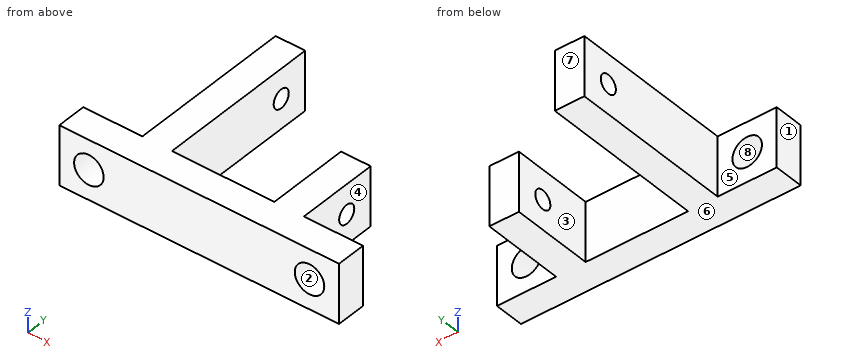
from build123d import *

# Parameters (mm, degrees)
SKETCH1_W           = 22.033357
SKETCH1_H           = 6.35
SKETCH1_W_2         = 12.7
BOSS_EXTRUDE1_DEPTH = 12.7
CUT_EXTRUDE1_REACH  = 49.433
SKETCH2_R           = 2
CUT_EXTRUDE2_REACH  = 8.35
SKETCH3_R           = 3.175
CUT_EXTRUDE3_REACH  = 49.433
SKETCH4_R           = 2


with BuildPart() as part:
    # Sketch1 → Boss-Extrude1 (new body)
    with BuildSketch(Plane.XY):
        Rectangle(SKETCH1_W, SKETCH1_H)
        Polygon((-11.0166785, -3.175), (-11.0166785, 3.175), (-11.0166785, 38.51148), (-17.3666785, 38.51148), (-17.3666785, 3.175), (-17.3666785, -3.175), align=None)
        Polygon((11.0166785, 20.87372), (11.0166785, 3.175), (11.0166785, -3.175), (17.3666785, -3.175), (17.3666785, 3.175), (17.3666785, 20.87372), align=None)
        with Locations((-23.7166785, 0)):
            Rectangle(SKETCH1_W_2, SKETCH1_H)
        with Locations((23.7166785, 0)):
            Rectangle(SKETCH1_W_2, SKETCH1_H)
    extrude(amount=BOSS_EXTRUDE1_DEPTH)

    # Sketch2 → Cut-Extrude1 (cut, up to next)
    with BuildSketch(Plane(origin=(17.3666785, 0, 0), x_dir=(0, 0, -1), z_dir=(1, 0, 0)), mode=Mode.PRIVATE) as cut_extrude1_sk1:
        with Locations((-6.35, 14.52372)):
            Circle(SKETCH2_R)
    cut_extrude1_tool1 = extrude(cut_extrude1_sk1.sketch, amount=-CUT_EXTRUDE1_REACH, mode=Mode.PRIVATE) & part.part
    add(cut_extrude1_tool1.solids().sort_by_distance((17.366678, 14.52372, 6.35))[0], mode=Mode.SUBTRACT)

    # Sketch3 → Cut-Extrude2 (cut, up to next)
    with BuildSketch(Plane(origin=(0, 3.175, 0), x_dir=(1, 0, 0), z_dir=(0, 1, 0)), mode=Mode.PRIVATE) as cut_extrude2_sk1:
        with Locations((-23.7166785, -6.35)):
            Circle(SKETCH3_R)
    cut_extrude2_tool1 = extrude(cut_extrude2_sk1.sketch, amount=-CUT_EXTRUDE2_REACH, mode=Mode.PRIVATE) & part.part
    add(cut_extrude2_tool1.solids().sort_by_distance((-23.716678, 3.175, 6.35))[0], mode=Mode.SUBTRACT)
    # Sketch3 → Cut-Extrude2 (cut, up to next)
    with BuildSketch(Plane(origin=(0, 3.175, 0), x_dir=(1, 0, 0), z_dir=(0, 1, 0)), mode=Mode.PRIVATE) as cut_extrude2_sk2:
        with Locations((23.7166785, -6.35)):
            Circle(SKETCH3_R)
    cut_extrude2_tool2 = extrude(cut_extrude2_sk2.sketch, amount=-CUT_EXTRUDE2_REACH, mode=Mode.PRIVATE) & part.part
    add(cut_extrude2_tool2.solids().sort_by_distance((23.716679, 3.175, 6.35))[0], mode=Mode.SUBTRACT)

    # Sketch4 → Cut-Extrude3 (cut, up to next)
    with BuildSketch(Plane.ZY.offset(17.3666785), mode=Mode.PRIVATE) as cut_extrude3_sk1:
        with Locations((6.35, 32.16148)):
            Circle(SKETCH4_R)
    cut_extrude3_tool1 = extrude(cut_extrude3_sk1.sketch, amount=-CUT_EXTRUDE3_REACH, mode=Mode.PRIVATE) & part.part
    add(cut_extrude3_tool1.solids().sort_by_distance((-17.366678, 32.16148, 6.35))[0], mode=Mode.SUBTRACT)


solid = part.part
For this review, take the finished solid that the model builds, in its own axes (mm). Face numbers are marked on the shaded views. A direction names the side the tool comes from. Coordinates: 2 decimals unless noted, no trailing zeros. Loops run counter-clockwise (first coordinate to the right, second up) from the corner with the lowest first, then second, coordinate; pieces in that order, holes last. Notation, with made-up numbers: (20.25, 65.5) - (71.25, 65.5) arc R22 ccw to (71.25, 99.5) - close; hole circle Ø3 at (77, 40). An arc over 180 degrees is marked (long way). Use a Markdown table: item, result. Add a question column.
Item 1: Tool access review of the marked faces 1, 2, 3, 4 and 5: name each direction out of +Z, -Z, +X, -X, +Y, -Y from which nothing blocks a thin tool from reaching the whole face with its end or side.
Item 2: We need section D-D (x = 4). Give the boundary of the cut face in (y, z) (3 decimals), and give its area (3 significant figures).
Item 3: We need section B-B (y = 18.5). Give the boundary of the cut face in (x, z).
Item 4: For line 1 (X direction, y = -1.5, z = 6.35); line 2 (Y direction, x = -14, z = 6.35) (3 decimals); line 3 (X direction, y = 1, z = 5.25), list the stretches that pass through material, from the lowest coordinate up.
Item 5: Insertion check: pin 1 Ø1.5 at (y, z) = (31, 9.5) entering from +X; pin 2 Ø7.5 at (x, z) = (-23.72, 6.35) entering from +Y (3 decimals); pin 3 Ø6.5 at (y, z) = (14, 6) entering from -X. Each pin has a flat end and moves straight along its axis. Give the tip position at first contact, or say it passes through.
Item 6: Mouldability with a two-part tool opening along Z and no side actions: class the marked faces 6, 7 and 8 as pulls with the +Z half, pulls with the -Z half, needs draft (parallel to the pull), parting line crosses it, or undercut.
Item 7: We need section C-C (z = 11). Give the boundary of the cut face in (x, y) (3 decimals).
Item 8: We need section A-A (z = 6.35). Give the boundary of the cut face in (x, y) (3 decimals), and give its area (3 significant figures).
Results list:
| question | item | result |
|---|---|---|
| 1 | face 1 | +Z, -Z, -X, +Y, -Y |
| 1 | face 2 | +Y, -Y |
| 1 | face 3 | +Z, -Z, +Y |
| 1 | face 4 | +Z, -Z, +X, +Y |
| 1 | face 5 | +Z, -Z, -X, +Y |
| 2 | outline | (-3.175, 0) - (3.175, 0) - (3.175, 12.7) - (-3.175, 12.7) - close |
| 2 | area | 80.6 mm^2 |
| 3 | outline | (-17.37, 0) - (-11.02, 0) - (-11.02, 12.7) - (-17.37, 12.7) - close; (11.02, 0) - (17.37, 0) - (17.37, 12.7) - (11.02, 12.7) - close |
| 4 | line 1 | x = -30.07 to -26.89, -20.54 to 20.54, 26.89 to 30.07 |
| 4 | line 2 | y = -3.175 to 30.161, 34.161 to 38.511 |
| 4 | line 3 | x = -30.07 to -26.7, -20.74 to 20.74, 26.7 to 30.07 |
| 5 | pin 1 | stops at x = -11.02 |
| 5 | pin 2 | stops at y = 3.175 |
| 5 | pin 3 | stops at x = -17.37 |
| 6 | face 6 | pulls with the -Z half |
| 6 | face 7 | needs draft |
| 6 | face 8 | undercut |
| 7 | outline | (-30.067, -3.175) - (30.067, -3.175) - (30.067, 3.175) - (17.367, 3.175) - (17.367, 20.874) - (11.017, 20.874) - (11.017, 3.175) - (-11.017, 3.175) - (-11.017, 38.511) - (-17.367, 38.511) - (-17.367, 3.175) - (-30.067, 3.175) - close |
| 8 | outline | (-30.067, -3.175) - (-26.892, -3.175) - (-26.892, 3.175) - (-30.067, 3.175) - close; (-20.542, -3.175) - (20.542, -3.175) - (20.542, 3.175) - (17.367, 3.175) - (17.367, 12.524) - (11.017, 12.524) - (11.017, 3.175) - (-11.017, 3.175) - (-11.017, 30.161) - (-17.367, 30.161) - (-17.367, 3.175) - (-20.542, 3.175) - close; (-17.367, 34.161) - (-11.017, 34.161) - (-11.017, 38.511) - (-17.367, 38.511) - close; (11.017, 16.524) - (17.367, 16.524) - (17.367, 20.874) - (11.017, 20.874) - close; (26.892, -3.175) - (30.067, -3.175) - (30.067, 3.175) - (26.892, 3.175) - close |
| 8 | area | 587 mm^2 |
